Input: part model. Units: mm. Frame: model coordinates. Face numbers are marked on the shaded views. A direction names the side the tool comes from. Give positions to 0.01 mm unless a question says otherwise; leave off trailing zeros. Order: outer loops, then holes, each group sorted by start corner. A loop starts at its lowest first (then second) coordinate and runs counter-clockwise, first axis right, second up. Notation, with made-up numbers: (56, 64.25) - (81, 64.25) arc R27 ccw to (81, 81.25) - close; hole circle Ø2 at (60.25, -36.5). An arc over 180 degrees is marked (long way). Use a Markdown table: item, result.
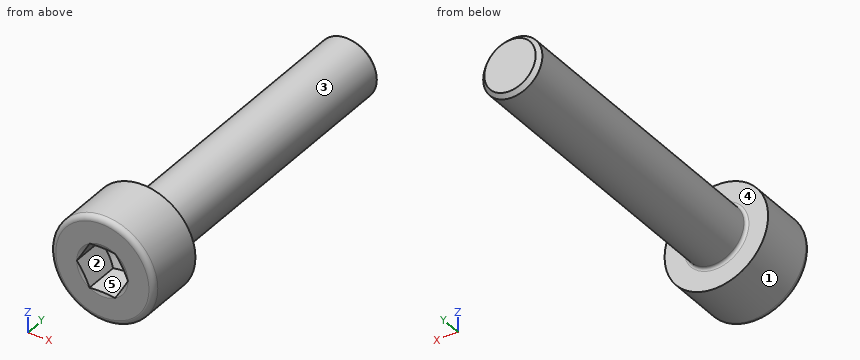
Solid Edge part; units mm, degrees
sketch "Sketch1" plane through (0, 0, 0) normal (0, 0, 1) x (1, 0, 0)
  line L0 (2, 0) -> (2, 20)
  line L1 (0, 20) -> (2, 20)
  line L2 (0, 0) -> (0, 20)
  line L3 (0, 0) -> (0, -4)
  line L4 (0, -4) -> (3.5, -4)
  line L5 (3.5, -4) -> (3.5, 0)
  line L6 (3.5, 0) -> (2, 0)
revolve "RevolvedProtrusion1" add sketch "Sketch1" angle 360 about axis through (0, 0, 0) along (0, 1, 0)
sketch "Sketch2" plane through (0, 0, 0) normal (1, 0, 0) x (0, 1, 0)
  line L0 (-4, 2.2215) -> (-2, 2.2215)
  line L1 (-0.7174, 0) -> (-2, 2.2215)
  line L2 (-4, 0) -> (-0.7174, 0)
  line L3 (-4, 0) -> (-4, 2.2215)
revolve "RevolvedCutout1" cut sketch "Sketch2" angle 360 about axis through (0, -4.5, 0) along (0, 1, 0)
sketch "Sketch3" plane through (0, -4, 0) normal (0, -1, 0) x (0, 0, 1)
  circle A0 centre (0, 0) radius 2.2215
  line L0 (-1.5, -0.866) -> (0, -1.7321)
  line L1 (0, -1.7321) -> (1.5, -0.866)
  line L2 (1.5, -0.866) -> (1.5, 0.866)
  line L3 (1.5, 0.866) -> (0, 1.7321)
  line L4 (0, 1.7321) -> (-1.5, 0.866)
  line L5 (-1.5, 0.866) -> (-1.5, -0.866)
extrude "Protrusion1" add sketch "Sketch3" against normal up to next
sketch "Sketch4" plane through (0, 0, 0) normal (0, 0, 1) x (1, 0, 0)
  line L0 (-1.7321, -4) -> (0, -4)
  line L1 (0, -4) -> (0, -3.5359)
  line L2 (0, -3.5359) -> (-1.7321, -4)
revolve "RevolvedCutout2" cut sketch "Sketch4" angle 360 about axis through (0, -4.5, 0) along (0, 1, 0)
fillet "Round1" radius 0.2 1 edges at (0, 0, -2)
fillet "Round2" radius 0.35 1 edges at (0, -4, -3.5)
chamfer "倒斜角_2" distance 0.2667 angle 45 1 edges at (0, 20, -2)
cosmetic_thread "螺纹_3" thread depth 16
1. Mould query, pull axis Z, two halves, no side actions, for the marked faces 3, 4 and 5. Classes: pulls with the +Z half, pulls with the -Z half, needs draft (parallel to the pull), parting line crosses it, or undercut.
Response:
| item | result |
|---|---|
| face 3 | parting line crosses it |
| face 4 | needs draft |
| face 5 | undercut |
2. Set-up query: the marked faces 1 and 2. Return all of +Z, -Z, +X, -X, +Y, -Y with unobstructed straight access to the full face (end or side cutting, diameter ignored); none if empty.
Response:
| item | result |
|---|---|
| face 1 | +Y, -Y |
| face 2 | -Y |
3. Material intervals for line 1 along Y through (x, z) = (-0.5, -2.25); line 2 along X through (y, z) = (-1.5, 0); line 3 along X through (y, z) = (2.75, 1.25), sorted ascending.
Response:
| item | result |
|---|---|
| line 1 | y = -4 to 0 |
| line 2 | x = -3.5 to -1.36, 1.36 to 3.5 |
| line 3 | x = -1.56 to 1.56 |
4. Pin query (flat end, axial travel): pin 1 (1.5 mm diameter, centred on y = 13, z = 2.5, fed in from -X); pin 2 (2 mm diameter, centred on x = 1.5, y = 4.5, fed in from +Z); pin 3 (1.5 mm diameter, centred on x = -2, y = 12, fed in from -Z). Return the tip coordinate at first contact, or that it passes through.
Response:
| item | result |
|---|---|
| pin 1 | stops at x = -0.97 |
| pin 2 | stops at z = 1.94 |
| pin 3 | stops at z = -1.56 |
5. Section query A-A (y = 7). Return loops of the section in (x, z).
Response:
| item | result |
|---|---|
| outline | circle Ø4 at (0, 0) |
